Part model, mm, in its own coordinate system. Face numbers are marked on the shaded views. A direction names the side the tool comes from. Round coordinates to 2 decimals unless told otherwise and drop trailing zeros. Order: outer loops, then holes, each group sorted by start corner. A loop starts at its lowest first (then second) coordinate and runs counter-clockwise, first axis right, second up. Notation, with made-up numbers: (62.25, 82) - (97.25, 82) arc R20 cw to (97.25, 98) - close; hole circle Ø10 at (18.5, 66.25). An arc over 180 degrees is marked (long way). Answer as a JSON object with one key per item and string values.
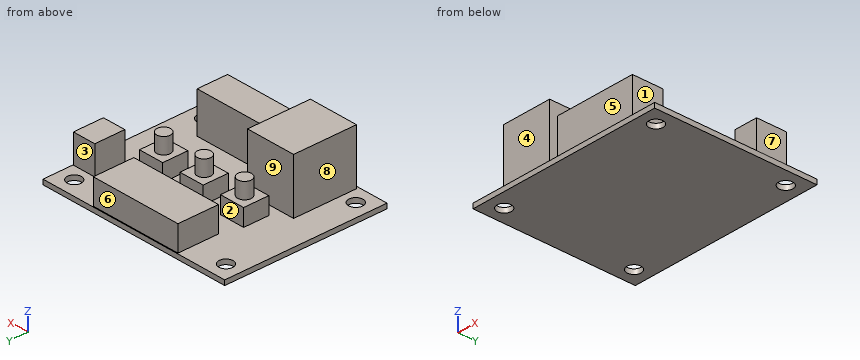
```python
from build123d import *

# Parameters (mm, degrees)
F0_W      = 48.5
F0_H      = 40
F0_R      = 1.75
F1_DEPTH  = 1.2
F2_W      = 22.6
F2_H      = 10
F3_DEPTH  = 6.2
F4_W      = 5.7
F4_H      = 7.4
F5_DEPTH  = 7
F6_W      = 20
F6_H      = 7.5
F7_DEPTH  = 10
F8_W      = 12.3
F8_H      = 15.5
F9_DEPTH  = 13.5
F10_W     = 6.2
F10_H     = 6.2
F10_R     = 1.7
F11_DEPTH = 4.2
F12_DEPTH = 8.1


with BuildPart() as f1:
    # F0 (on Top) → F1 (new body)
    with BuildSketch(Plane.XY):
        Rectangle(F0_W, F0_H)
        with Locations((-20.25, -16)):
            Circle(F0_R, mode=Mode.SUBTRACT)
        with Locations((20.25, -16)):
            Circle(F0_R, mode=Mode.SUBTRACT)
        with Locations((-20.25, 16)):
            Circle(F0_R, mode=Mode.SUBTRACT)
        with Locations((20.25, 16)):
            Circle(F0_R, mode=Mode.SUBTRACT)
    extrude(amount=F1_DEPTH)

    # F2 (on face) → F3 (join)
    with BuildSketch(Plane.XY.offset(1.2)):
        with Locations((-0.25, 14.8)):
            Rectangle(F2_W, F2_H)
    extrude(amount=F3_DEPTH)

    # F4 (on face) → F5 (join)
    with BuildSketch(Plane.XY.offset(1.2)):
        with Locations((21.3, 8.9)):
            Rectangle(F4_W, F4_H)
    extrude(amount=F5_DEPTH)

    # F6 (on face) → F7 (join)
    with BuildSketch(Plane.XY.offset(1.2)):
        with Locations((6.45, -14.55)):
            Rectangle(F6_W, F6_H)
    extrude(amount=F7_DEPTH)

    # F8 (on face) → F9 (join)
    with BuildSketch(Plane.XY.offset(1.2)):
        with Locations((-10.6, -11.65)):
            Rectangle(F8_W, F8_H)
    extrude(amount=F9_DEPTH)

    # F10 (on face) → F11 (join)
    with BuildSketch(Plane.XY.offset(1.2)):
        with Locations((11.75, 1.8)):
            Rectangle(F10_W, F10_H)
        with Locations((11.75, 1.8)):
            Circle(F10_R, mode=Mode.SUBTRACT)
        with Locations((0.95, 1.8)):
            Rectangle(F10_W, F10_H)
        with Locations((0.95, 1.8)):
            Circle(F10_R, mode=Mode.SUBTRACT)
        with Locations((-9.85, 1.8)):
            Rectangle(F10_W, F10_H)
        with Locations((-9.85, 1.8)):
            Circle(F10_R, mode=Mode.SUBTRACT)
    extrude(amount=F11_DEPTH)

    # F12 (add): faces of the model
    f12_faces = [f1.faces().sort_by_distance(p)[0] for p in [
        (-9.85, 1.8, 1.2),
        (0.95, 1.8, 1.2),
        (11.75, 1.8, 1.2),
    ]]
    extrude(f12_faces, amount=F12_DEPTH)


solid = f1.part
```
Item 1: Drop flat-ended pins along their axis: P1, Ø2, axis at x = -4.5, z = 5.5, coming from the -Y side; P2, Ø4, axis at y = -6, z = 12, coming from the +X side; P3, Ø3, axis at x = 7.5, z = 4, coming from the -Y side. Give the stop position or say it passes through.
Taken from the geometry:
{"P1": "y = -19.4", "P2": "x = -4.45", "P3": "y = -18.3"}
Item 2: Cut at A-A (x = 20.25). Write the cut outline in (y, z).
Taken from the geometry:
{"outline": "(-20, 0) - (-17.75, 0) - (-17.75, 1.2) - (-20, 1.2) - close; (-14.25, 0) - (14.25, 0) - (14.25, 1.2) - (12.6, 1.2) - (12.6, 8.2) - (5.2, 8.2) - (5.2, 1.2) - (-14.25, 1.2) - close; (17.75, 0) - (20, 0) - (20, 1.2) - (17.75, 1.2) - close"}
Item 3: Probe L1, parallel to Y at x = 20.25, z = 0.55; L2, parallel to Y at x = 2.5, z = 3.5; L3, parallel to Y at x = 6.5, z = 4. List the from-to ranges inside material, lowest first. Write a range as from..to.
Taken from the geometry:
{"L1": "-20..-17.75, -14.25..14.25, 17.75..20", "L2": "-18.3..-10.8, -1.3..4.9, 9.8..19.8", "L3": "-18.3..-10.8, 9.8..19.8"}
Item 4: Two-plate mould, pull along Y, no slides. Class the marked faces 1, 2, 3 and 4: pulls with the +Y half, pulls with the -Y half, needs draft (parallel to the pull), parting line crosses it, or undercut.
Taken from the geometry:
{"face 1": "needs draft", "face 2": "undercut", "face 3": "pulls with the +Y half", "face 4": "pulls with the -Y half"}
Item 5: Tool access for the marked faces 5, 6, 7, 8 and 9: list every direction of +Z, -Z, +X, -X, +Y, -Y with a clear straight run to the whole face (end or side of a thin tool).
Taken from the geometry:
{"face 5": "+Z, +X, -Y", "face 6": "+Z, +X, -X, +Y", "face 7": "+Z, +X, +Y, -Y", "face 8": "+Z, -X, +Y, -Y", "face 9": "+Z, +X, -X"}
Item 6: Cut at C-C (z = 4.75). Write the cut outline in (x, y), plus the area to 3 significant figures.
Taken from the geometry:
{"outline": "(-16.75, -19.4) - (-4.45, -19.4) - (-4.45, -3.9) - (-16.75, -3.9) - close; (-12.95, -1.3) - (-6.75, -1.3) - (-6.75, 4.9) - (-12.95, 4.9) - close; (-11.55, 9.8) - (11.05, 9.8) - (11.05, 19.8) - (-11.55, 19.8) - close; (-3.55, -18.3) - (16.45, -18.3) - (16.45, -10.8) - (-3.55, -10.8) - close; (-2.15, -1.3) - (4.05, -1.3) - (4.05, 4.9) - (-2.15, 4.9) - close; (8.65, -1.3) - (14.85, -1.3) - (14.85, 4.9) - (8.65, 4.9) - close; (18.45, 5.2) - (24.15, 5.2) - (24.15, 12.6) - (18.45, 12.6) - close", "area": "724 mm2"}
Item 7: Cut at D-D (y = 1.8). Write the cut outline in (x, z).
Taken from the geometry:
{"outline": "(-24.25, 0) - (24.25, 0) - (24.25, 1.2) - (14.85, 1.2) - (14.85, 5.4) - (13.45, 5.4) - (13.45, 9.3) - (10.05, 9.3) - (10.05, 5.4) - (8.65, 5.4) - (8.65, 1.2) - (4.05, 1.2) - (4.05, 5.4) - (2.65, 5.4) - (2.65, 9.3) - (-0.75, 9.3) - (-0.75, 5.4) - (-2.15, 5.4) - (-2.15, 1.2) - (-6.75, 1.2) - (-6.75, 5.4) - (-8.15, 5.4) - (-8.15, 9.3) - (-11.55, 9.3) - (-11.55, 5.4) - (-12.95, 5.4) - (-12.95, 1.2) - (-24.25, 1.2) - close"}
Item 8: Cut at B-B (y = 16). Write the cut outline in (x, z), plus the area to 3 significant figures.
Taken from the geometry:
{"outline": "(-24.25, 0) - (-22, 0) - (-22, 1.2) - (-24.25, 1.2) - close; (-18.5, 0) - (18.5, 0) - (18.5, 1.2) - (11.05, 1.2) - (11.05, 7.4) - (-11.55, 7.4) - (-11.55, 1.2) - (-18.5, 1.2) - close; (22, 0) - (24.25, 0) - (24.25, 1.2) - (22, 1.2) - close", "area": "190 mm2"}
